Design review of the part built by this model. Coordinates are the model's own, in mm. Face numbers are marked on the shaded views. A direction names the side the tool comes from. Give positions to 0.01 mm unless a question says otherwise; leave off trailing zeros. Write each loop counter-clockwise with the first axis right and the second up, starting at its lowest first coordinate (ties: lowest second). Pieces come first, ordered by that corner, then holes. Notation, with made-up numbers: (56.25, 39) -> (98.25, 39) arc R24 ccw to (98.25, 70) -> close; hole circle Ø1 at (52, 80). An arc over 180 degrees is marked (long way). Put each result on its own line as item: value. Start each with the question number.
from build123d import *

# Parameters (mm, degrees)
SKETCH_1_R      = 5
EXTRUDE_1_DEPTH = 10
DRAFT_1_ANGLE   = 15
SKETCH_3_R      = 7.679492
EXTRUDE_2_DEPTH = 10
DRAFT_2_ANGLE   = -15


with BuildPart() as part:
    # Эскиз1 → Вытянуть1 (new body)
    with BuildSketch(Plane(origin=(0, 0, 0), x_dir=(1, 0, 0), z_dir=(0, 1, 0))):
        with Locations(Location((0, 0, 0), (0, 0, 270))):
            Circle(SKETCH_1_R)
        with BuildLine():
            Line((2, 1.5), (2, -1.5))
            ThreePointArc((2, -1.5), (-2.5, 0), (2, 1.5))
        make_face(mode=Mode.SUBTRACT)
    extrude(amount=EXTRUDE_1_DEPTH)

    # Уклон1
    draft_1_faces = [part.faces().sort_by_distance(p)[0] for p in [
        (0, 5, -5),
    ]]
    draft(draft_1_faces, Plane.ZX.offset(10), DRAFT_1_ANGLE)

    # Эскиз3 → Вытянуть2 (add)
    with BuildSketch(Plane(origin=(0, 10, 0), x_dir=(1, 0, 0), z_dir=(0, 1, 0))):
        with Locations(Location((0, 0, 0), (0, 0, 270))):
            Circle(SKETCH_3_R)
        with BuildLine():
            Line((2, 1.5), (2, -1.5))
            ThreePointArc((2, -1.5), (-2.5, 0), (2, 1.5))
        make_face(mode=Mode.SUBTRACT)
    extrude(amount=EXTRUDE_2_DEPTH)

    # Уклон2
    draft_2_faces = [part.faces().sort_by_distance(p)[0] for p in [
        (0, 15, -7.679492),
    ]]
    draft(draft_2_faces, Plane.ZX.offset(20), DRAFT_2_ANGLE)


solid = part.part
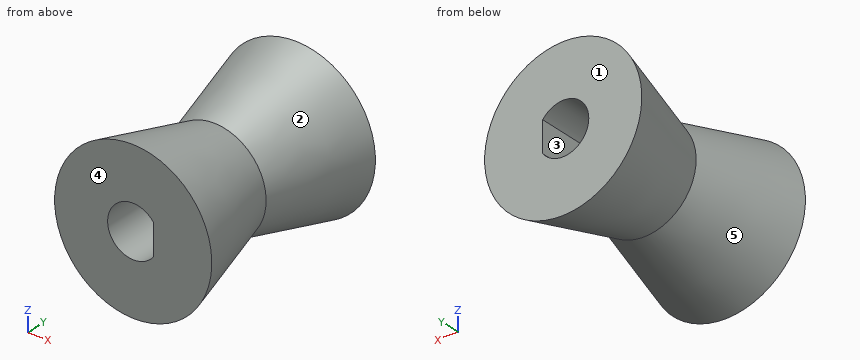
Q1. For pin 1 (2.5 mm diameter, centred on y = 5.5, z = 0, fed in from -X); pin 2 (1.5 mm diameter, centred on y = 7.5, z = 4, fed in from -X), all flat-tipped, find the tip position at first contact; note any pin that passes through.
Q2. Machinability: for the marked faces 4 and 5, which of the approach directions +Z, -Z, +X, -X, +Y, -Y give a long, thin tool a straight path to every point of the face, cutting with its end or side? Answer none if there is none.
Q3. Take a section at C-C on y = 11.25. Give the boundary of the cut face in (x, z).
Q4. Take a section at B-B on y = 5. Give the boundary of the cut face in (x, z).
Q5. Mouldability with a two-part tool opening along X and no side actions: class the marked faces 1, 2 and 3 as +X half, -X half, draft (parallel to the pull), parting line (faces both ways), or undercut.
Q6. To check wall thickness, follow probe 1 along Z at (x, y) = (0, 12.5); probe 2 along Z at (x, y) = (0, 8); probe 3 along X at (y, z) = (13.25, 0). State the ranges of each line that lie inside material, in increasing order. Write a range as from..to.
Result:
1. pin 1: stops at x = -6.54
1. pin 2: stops at x = -4.7
2. face 4: +Z, -Z, +X, -X, -Y
2. face 5: none
3. outline: circle Ø10.67 at (0, 0); hole (2, -1.5) -> (2, 1.5) arc R2.5 ccw (long way) to start
4. outline: circle Ø12.68 at (0, 0); hole (2, -1.5) -> (2, 1.5) arc R2.5 ccw (long way) to start
5. face 1: draft
5. face 2: parting line
5. face 3: undercut
6. probe 1: z = -5.67..-2.5, 2.5..5.67
6. probe 2: z = -5.54..-2.5, 2.5..5.54
6. probe 3: x = -5.87..-2.5, 2..5.87
